Read the model definition and answer for the solid it produces. Units are mm, in the model's axes. A direction names the side the tool comes from. Coordinates: 2 decimals unless noted, no trailing zeros. Loops run counter-clockwise (first coordinate to the right, second up) from the corner with the lowest first, then second, coordinate; pieces in that order, holes last. Notation, with made-up numbers: (1.25, 79) -> (27.25, 79) arc R13 cw to (27.25, 85) -> close; hole circle Ø9 at (29, 38.25). An arc over 180 degrees is marked (long way). One line per question, with ' | ' between items. Start each with the question number.
```python
from build123d import *

# Parameters (mm, degrees)
SKETCH1_R              = 2.54
SKETCH1_R_2            = 6.35
MAINBASEPLATE_DEPTH    = 3
PANTILT_EXTRUDE6_DEPTH = 53.34
SKETCH11_W             = 69.5
SKETCH11_H             = 37.75
BOSS_EXTRUDE7_DEPTH    = 3
SKETCH12_R             = 2.0193
CUT_EXTRUDE3_DEPTH     = 56.34
SKETCH32_W             = 712.395528774
SKETCH32_H             = 524.196017535
CUT_EXTRUDE11_DEPTH    = 3
SKETCH33_W             = 30
SKETCH33_H             = 10
SKETCH33_R             = 2.5
BOSS_EXTRUDE9_DEPTH    = 2.5
FILLET1_R              = 2


with BuildPart() as part:
    # Sketch1 → mainbaseplate (new body)
    with BuildSketch(Plane(origin=(0, 0, 0), x_dir=(1, 0, 0), z_dir=(0, 1, 0))):
        with BuildLine():
            Line((-223.52, -111.125), (223.52, -111.125))
            ThreePointArc((223.52, -111.125), (227.112102448, -109.637102448), (228.6, -106.045))
            Line((228.6, -106.045), (228.6, 106.045))
            ThreePointArc((228.6, 106.045), (227.112102448, 109.637102448), (223.52, 111.125))
            Line((223.52, 111.125), (-223.52, 111.125))
            ThreePointArc((-223.52, 111.125), (-227.112102448, 109.637102448), (-228.6, 106.045))
            Line((-228.6, 106.045), (-228.6, -106.045))
            ThreePointArc((-228.6, -106.045), (-227.112102448, -109.637102448), (-223.52, -111.125))
        make_face()
        with Locations(Location((127, 36.5125, 0), (0, 0, 270))):
            Circle(SKETCH1_R, mode=Mode.SUBTRACT)
        with Locations(Location((127, -36.5125, 0), (0, 0, 270))):
            Circle(SKETCH1_R, mode=Mode.SUBTRACT)
        with Locations(Location((-142.24, 36.5125, 0), (0, 0, 270))):
            Circle(SKETCH1_R, mode=Mode.SUBTRACT)
        with Locations(Location((-142.24, -36.5125, 0), (0, 0, 270))):
            Circle(SKETCH1_R, mode=Mode.SUBTRACT)
        with Locations(Location((209.55, 0, 0), (0, 0, 270))):
            Circle(SKETCH1_R_2, mode=Mode.SUBTRACT)
    extrude(amount=MAINBASEPLATE_DEPTH)

    # Sketch10 → PanTilt-Extrude6 (add)
    with BuildSketch(Plane(origin=(0, 3, 0), x_dir=(1, 0, 0), z_dir=(0, 1, 0))):
        Polygon((104.95, 18.875), (174.45, 18.875), (174.45, -18.875), (104.95, -18.875), (104.95, -6.175), (107.95, -6.175), (107.95, -15.875), (171.45, -15.875), (171.45, 15.875), (107.95, 15.875), (107.95, 6.175), (104.95, 6.175), align=None)
    extrude(amount=PANTILT_EXTRUDE6_DEPTH)

    # Sketch11 → Boss-Extrude7 (add)
    with BuildSketch(Plane(origin=(0, 56.34, 0), x_dir=(1, 0, 0), z_dir=(0, 1, 0))):
        with Locations((139.7, 0)):
            Rectangle(SKETCH11_W, SKETCH11_H)
    extrude(amount=BOSS_EXTRUDE7_DEPTH)

    # Sketch12 → Cut-Extrude3 (cut)
    with BuildSketch(Plane(origin=(0, 59.34, 0), x_dir=(1, 0, 0), z_dir=(0, 1, 0))):
        with Locations(Location((163.83, 5.08, 0), (0, 0, 270))):
            Circle(SKETCH12_R)
        with Locations(Location((163.83, -5.08, 0), (0, 0, 270))):
            Circle(SKETCH12_R)
        with Locations(Location((115.57, 5.08, 0), (0, 0, 270))):
            Circle(SKETCH12_R)
        with Locations(Location((115.57, -5.08, 0), (0, 0, 270))):
            Circle(SKETCH12_R)
        Polygon((118.745, 1.937698292), (104.95, 1.937698292), (95.841621454, 0), (104.95, -1.990085687), (118.745, -1.990085687), (118.745, -10.795), (160.655, -10.795), (160.655, 10.795), (118.745, 10.795), align=None)
    extrude(amount=-CUT_EXTRUDE3_DEPTH, mode=Mode.SUBTRACT)

    # Sketch32 → Cut-Extrude11 (cut)
    with BuildSketch(Plane.XZ):
        with Locations((-5.907824988, 36.768742763)):
            Rectangle(SKETCH32_W, SKETCH32_H)
    extrude(amount=-CUT_EXTRUDE11_DEPTH, mode=Mode.SUBTRACT)

    # Sketch33 → Boss-Extrude9 (add)
    # profile 1 of 2: a face of its own
    with BuildSketch(Plane.XZ.offset(-3)):
        with Locations((139.7, 23.875)):
            Rectangle(SKETCH33_W, SKETCH33_H)
        with Locations(Location((132.2, 23.875, 0), (0, 0, 270))):
            Circle(SKETCH33_R, mode=Mode.SUBTRACT)
        with Locations(Location((147.2, 23.875, 0), (0, 0, 270))):
            Circle(SKETCH33_R, mode=Mode.SUBTRACT)
    # profile 2 of 2: a face of its own
    with BuildSketch(Plane.XZ.offset(-3)):
        with Locations((139.7, -23.875)):
            Rectangle(SKETCH33_W, SKETCH33_H)
        with Locations(Location((132.2, -23.875, 0), (0, 0, 270))):
            Circle(SKETCH33_R, mode=Mode.SUBTRACT)
        with Locations(Location((147.2, -23.875, 0), (0, 0, 270))):
            Circle(SKETCH33_R, mode=Mode.SUBTRACT)
    extrude(amount=-BOSS_EXTRUDE9_DEPTH)

    # Fillet1
    fillet1_edges = [part.edges().sort_by_distance(p)[0] for p in [
        (124.7, 4.25, 28.875),
        (154.7, 4.25, 28.875),
        (154.7, 4.25, 18.875),
        (124.7, 4.25, 18.875),
        (139.7, 5.5, 18.875),
        (124.7, 4.25, -18.875),
        (154.7, 4.25, -18.875),
        (154.7, 4.25, -28.875),
        (124.7, 4.25, -28.875),
        (139.7, 5.5, -18.875),
    ]]
    fillet(fillet1_edges, radius=FILLET1_R)


solid = part.part
```
(1) Section A-A on x = 115.57 is taken. Write down the section's boundary in (y, z) (3 decimals).
(2) Section B-B on z = -13.5 is taken. Write down the section's boundary in (x, y).
(3) A tool of negligible diameter and unlimited length cuts with its end or side. For faces 5 (the flat face through (118.745, 58, 6)), 6 (the flat face through (124.7, 4, 24)), 7 (the flat face through (140, 29, -15.875)), from which of +Z, -Z, +X, -X, +Y, -Y can it reach the whole face along a straight path? Write none if from no direction.
(4) Find the intervals of material crossed by probe 1 along X at (y, z) = (58.3, 5.08) (3 decimals); probe 2 along Z at (x, y) = (163.83, 58.3) (3 decimals); probe 3 along Z at (x, y) = (132.2, 5) (3 decimals), in increasing order. Write a range as from..to.
(5) Section C-C on x = 136.5 is taken. Write down the section's boundary in (y, z) (3 decimals), plus the area to 3 significant figures.
(6) Each of these flat-tipped pins is pushed along its axis until it touches: pin 1 Ø0.8 at (y, z) = (4.5, 23) entering from +X; pin 2 Ø5.5 at (x, z) = (115.57, 5.08) entering from -Y; pin 3 Ø4 at (x, y) = (125, 28) entering from -Z (3 decimals); pin 4 Ø4.5 at (x, z) = (147.2, 23.875) entering from -Y. Where does it stop, or does it pass through?
(7) Determine the mould class of faces 1 (the cylindrical face through (154.13, 4.268, -28.274)), 2 (the cylindrical face through (123.829, 4.782, 19.224)), 3 (the flat face through (106, 29, -6.175)), 4 (the flat face through (140, 3, -17)) for opening direction Z: +Z half, -Z half, draft (parallel to the pull), parting line (faces both ways), or undercut.
(8) Section D-D on y = 23.5 is taken. Write down the section's boundary in (x, z) (3 decimals), plus the area to 3 significant figures.
Working result:
1) outline: (3, -18.875) -> (59.34, -18.875) -> (59.34, -7.099) -> (56.34, -7.099) -> (56.34, -15.875) -> (3, -15.875) -> close; (3, 15.875) -> (56.34, 15.875) -> (56.34, 7.099) -> (59.34, 7.099) -> (59.34, 18.875) -> (3, 18.875) -> close; (56.34, -3.061) -> (59.34, -3.061) -> (59.34, -1.938) -> (56.34, -1.938) -> close; (56.34, 1.99) -> (59.34, 1.99) -> (59.34, 3.061) -> (56.34, 3.061) -> close
2) outline: (104.95, 3) -> (107.95, 3) -> (107.95, 56.34) -> (171.45, 56.34) -> (171.45, 3) -> (174.45, 3) -> (174.45, 59.34) -> (104.95, 59.34) -> close
3) face 5: +Y, -Y | face 6: +Z, -X, +Y, -Y | face 7: -Y
4) probe 1: x = 104.95..113.551, 117.589..118.745, 160.655..161.811, 165.849..174.45 | probe 2: z = -18.875..-7.099, -3.061..3.061, 7.099..18.875 | probe 3: z = -28.875..-26.375, -21.375..-15.875, 15.875..21.375, 26.375..28.875
5) outline: (3, -28.875) -> (5.5, -28.875) -> (5.5, -20.875) arc R2 cw to (7.5, -18.875) -> (59.34, -18.875) -> (59.34, -10.795) -> (56.34, -10.795) -> (56.34, -15.875) -> (3, -15.875) -> close; (3, 15.875) -> (56.34, 15.875) -> (56.34, 10.795) -> (59.34, 10.795) -> (59.34, 18.875) -> (7.5, 18.875) arc R2 cw to (5.5, 20.875) -> (5.5, 28.875) -> (3, 28.875) -> close | area: 420 mm2
6) pin 1: stops at x = 154.7 | pin 2: stops at y = 56.34 | pin 3: stops at z = -18.875 | pin 4: passes through
7) face 1: -Z half | face 2: +Z half | face 3: undercut | face 4: draft
8) outline: (104.95, -18.875) -> (174.45, -18.875) -> (174.45, 18.875) -> (104.95, 18.875) -> (104.95, 6.175) -> (107.95, 6.175) -> (107.95, 15.875) -> (171.45, 15.875) -> (171.45, -15.875) -> (107.95, -15.875) -> (107.95, -6.175) -> (104.95, -6.175) -> close | area: 570 mm2
